Here's how the part is built. I have some questions about the finished solid (model axes, mm). Face numbers are marked on the shaded views. A direction names the side the tool comes from. Round coordinates to 2 decimals unless told otherwise and drop trailing zeros. Loops run counter-clockwise (first coordinate to the right, second up) from the corner with the lowest first, then second, coordinate; pieces in that order, holes last. Notation, with made-up numbers: M 51.5,-14 L 103.5,-14 A7 ccw 103.5,-6 Z; hole C 75.5,-4.5 d8. An arc over 180 degrees is marked long. Answer as a JSON object with one key per item and string values.
from build123d import *

# Parameters (mm, degrees)
SKETCH_1_W          = 100
SKETCH_1_H          = 40
EXTRUDE_1_DEPTH     = 20
SKETCH_2_W          = 96
SKETCH_2_H          = 36
CUT_EXTRUDE_1_DEPTH = 10
SKETCH_3_W          = 80.4
SKETCH_3_H          = 20
EXTRUDE_2_DEPTH     = 27.2
CUT_EXTRUDE_2_DEPTH = 27.2
FILLET_1_R          = 1


with BuildPart() as part:
    # Эскиз1 → Бобышка-Вытянуть1 (new body)
    with BuildSketch(Plane.XY):
        Rectangle(SKETCH_1_W, SKETCH_1_H)
    extrude(amount=EXTRUDE_1_DEPTH)

    # Эскиз2 → Вырез-Вытянуть1 (cut)
    with BuildSketch(Plane.XY.offset(20)):
        Rectangle(SKETCH_2_W, SKETCH_2_H)
    extrude(amount=-CUT_EXTRUDE_1_DEPTH, mode=Mode.SUBTRACT)

    # Эскиз3 → Бобышка-Вытянуть2 (add)
    with BuildSketch(Plane(origin=(0, 20, 0), x_dir=(1, 0, 0), z_dir=(0, 1, 0))):
        with Locations((0, -10)):
            Rectangle(SKETCH_3_W, SKETCH_3_H)
    extrude(amount=EXTRUDE_2_DEPTH)

    # Эскиз4 → Вырез-Вытянуть2 (cut)
    with BuildSketch(Plane.XZ.offset(-18)):
        Polygon((-38.2, 20), (0, 20), (38.2, 20), (38.2, 10), (-38.2, 10), align=None)
    extrude(amount=-CUT_EXTRUDE_2_DEPTH, mode=Mode.SUBTRACT)

    # Скругление1
    fillet_1_edges = [part.edges().sort_by_distance(p)[0] for p in [
        (50, 0, 20),
        (45.1, 20, 20),
        (-45.1, 20, 0),
        (-45.1, 20, 20),
        (-40.2, 33.6, 20),
        (40.2, 20, 10),
        (40.2, 33.6, 20),
        (40.2, 33.6, 0),
        (-40.2, 20, 10),
        (-40.2, 33.6, 0),
        (0, 47.2, 20),
        (40.2, 47.2, 10),
        (0, 47.2, 0),
        (-40.2, 47.2, 10),
        (-50, 0, 20),
        (45.1, 20, 0),
        (50, 0, 0),
        (0, -20, 0),
        (-50, 0, 0),
        (-50, 20, 10),
        (50, 20, 10),
        (50, -20, 10),
        (-50, -20, 10),
        (0, -20, 20),
    ]]
    fillet(fillet_1_edges, radius=FILLET_1_R)


solid = part.part
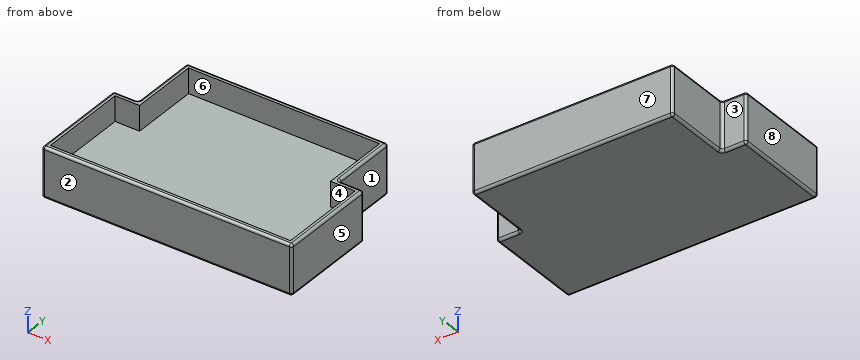
Item 1: For P1, Ø11, axis at y = 33, z = 16.5, coming from the +X side; P2, Ø11, axis at y = 35.5, z = 12.5, coming from the -X side; P3, Ø10, axis at x = 31, y = -9, coming from the +Z side, each with a flat end and sliding along its axis, tell me the tip position at first contact or that it passes through.
Solution:
{"P1": "stops at x = 40.2", "P2": "stops at x = -40.2", "P3": "stops at z = 10"}
Item 2: We'd pull the mould along Y, two halves only. Please class the marked faces 6, 7 and 8: +Y half, -Y half, draft (parallel to the pull), parting line (faces both ways), or undercut.
Solution:
{"face 6": "undercut", "face 7": "+Y half", "face 8": "draft"}
Item 3: I want a section at D-D on x = 7. List the corners of the cut face in (y, z) for me, plus the area to 3 significant figures.
Solution:
{"outline": "M -20,1 A1 ccw -19,0 L 46.2,0 A1 ccw 47.2,1 L 47.2,19 A1 ccw 46.2,20 L 45.2,20 L 45.2,10 L -18,10 L -18,20 L -19,20 A1 ccw -20,19 Z", "area": "711 mm2"}
Item 4: I want a section at A-A on z = 14.5. List the corners of the cut face in (x, y) for me, plus the area to 3 significant figures.
Solution:
{"outline": "M -50,-19 A1 ccw -49,-20 L 49,-20 A1 ccw 50,-19 L 50,19 A1 ccw 49,20 L 41.2,20 A1 cw 40.2,21 L 40.2,46.2 A1 ccw 39.2,47.2 L -39.2,47.2 A1 ccw -40.2,46.2 L -40.2,21 A1 cw -41.2,20 L -49,20 A1 ccw -50,19 Z; hole M -48,-18 L 48,-18 L 48,18 L 38.2,18 L 38.2,45.2 L -38.2,45.2 L -38.2,18 L -48,18 Z", "area": "652 mm2"}
Item 5: For the marked faces 1, 2, 3, 4 and 5, which set-ups out of +Z, -Z, +X, -X, +Y, -Y let a thin tool reach every point of the face, with its end or its side?
Solution:
{"face 1": "+Z, -Z, +X, +Y", "face 2": "+Z, -Z, +X, -X, -Y", "face 3": "+Z, -Z, -X, +Y", "face 4": "+Z", "face 5": "+Z, -Z, +X, +Y, -Y"}
Item 6: I want a section at C-C on y = 26.5. List the corners of the cut face in (x, z) for me, plus the area to 3 significant figures.
Solution:
{"outline": "M -40.2,1 A1 ccw -39.2,0 L 39.2,0 A1 ccw 40.2,1 L 40.2,19 A1 ccw 39.2,20 L 38.2,20 L 38.2,10 L -38.2,10 L -38.2,20 L -39.2,20 A1 ccw -40.2,19 Z", "area": "843 mm2"}
Item 7: I want a section at B-B on z = 4. List the corners of the cut face in (x, y) for me, plus the area to 3 significant figures.
Solution:
{"outline": "M -50,-19 A1 ccw -49,-20 L 49,-20 A1 ccw 50,-19 L 50,19 A1 ccw 49,20 L 41.2,20 A1 cw 40.2,21 L 40.2,46.2 A1 ccw 39.2,47.2 L -39.2,47.2 A1 ccw -40.2,46.2 L -40.2,21 A1 cw -41.2,20 L -49,20 A1 ccw -50,19 Z", "area": "6,190 mm2"}
Item 8: If I drill on L1, parallel to X at y = -4, z = 17; L2, parallel to Y at x = -34, z = 14.25; L3, parallel to Y at x = 41, z = 14.25, over which ranges is the centre line in solid material (lowest first)? Write a range as from..to.
Solution:
{"L1": "x = -50..-48, 48..50", "L2": "y = -20..-18, 45.2..47.2", "L3": "y = -20..-18, 18..20.02"}
